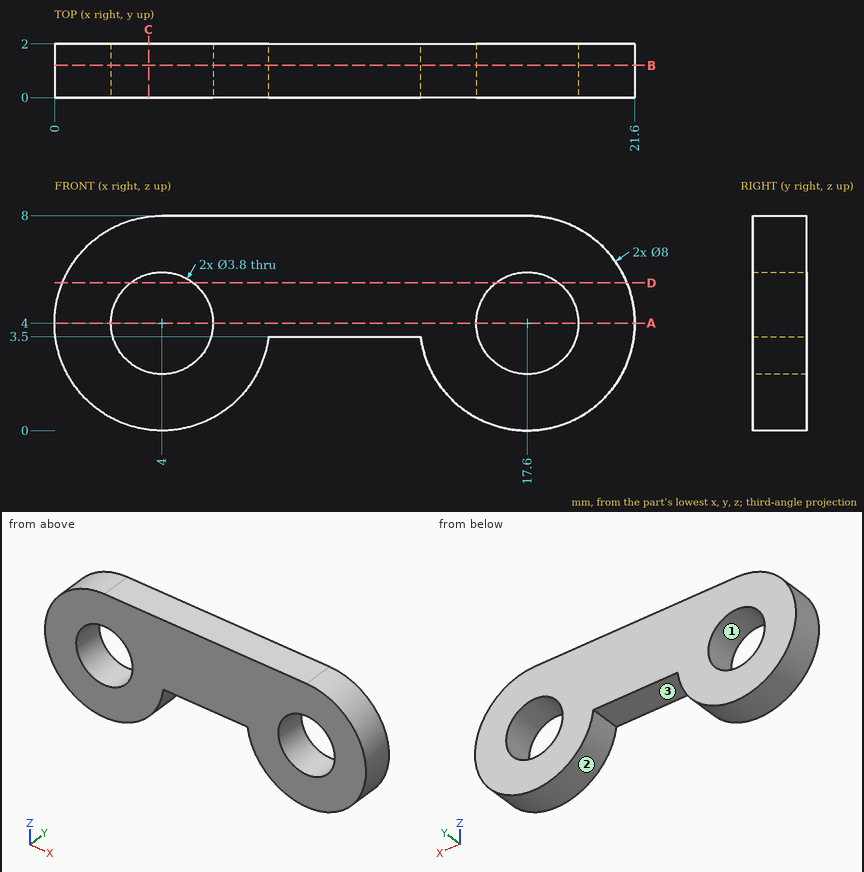
Can you work these out from the drawing? Everything is in mm from the part's minimum corner. Coordinates: 2 decimals unless noted, no trailing zeros. Loops run counter-clockwise (first coordinate to the right, second up) from the corner with the lowest first, then second, coordinate; pieces in that order, holes last. Notation, with made-up numbers: (41, 40.25) - (98, 40.25) arc R7 ccw to (98, 46.25) - close; hole circle Ø11 at (64.5, 33.5). An arc over 180 degrees is marked (long way). Put each result on its own line as item: value. Start each with the question number.
Item 1: Suppose I cut it at D-D (z = 5.5). Please give me the cut outline in (x, y).
Item 2: Suppose I cut it at A-A (z = 4). Please give me the cut outline in (x, y), and give its area (3 significant figures).
Item 3: If I drill on line 1 along X through (y, z) = (0.75, 4); line 2 along X through (y, z) = (1.5, 3.25); line 3 along X through (y, z) = (1.05, 5), over which ranges is the centre line in solid material (lowest first)?
Item 4: Suppose I cut it at C-C (x = 3.5). Please give me the cut outline in (y, z), and give its area (3 significant figures).
Item 5: For pin 1 (1 mm diameter, centred on y = 1.5, z = 1.5, fed in from -X), with a flat end and sliding along its axis, tell me the tip position at first contact or that it passes through.
Item 6: Suppose I cut it at B-B (y = 1.2). Please give me the cut outline in (x, z), and give its area (3 significant figures).
Item 7: If we mould it in two halves opening along Z, with no side actions, what happens to the marked faces 1, 2 and 3? For each: +Z half, -Z half, draft (parallel to the pull), parting line (faces both ways), or undercut.
Here are the results:
1. outline: (0.29, 0) - (2.83, 0) - (2.83, 2) - (0.29, 2) - close; (5.17, 0) - (16.43, 0) - (16.43, 2) - (5.17, 2) - close; (18.77, 0) - (21.31, 0) - (21.31, 2) - (18.77, 2) - close
2. outline: (0, 0) - (2.1, 0) - (2.1, 2) - (0, 2) - close; (5.9, 0) - (15.7, 0) - (15.7, 2) - (5.9, 2) - close; (19.5, 0) - (21.6, 0) - (21.6, 2) - (19.5, 2) - close
2. area: 28.0 mm²
3. line 1: 0 to 2.1, 5.9 to 15.7, 19.5 to 21.6
3. line 2: 0.07 to 2.25, 5.75 to 7.93, 13.67 to 15.85, 19.35 to 21.53
3. line 3: 0.13 to 2.38, 5.62 to 15.98, 19.22 to 21.47
4. outline: (0, 0.03) - (2, 0.03) - (2, 2.17) - (0, 2.17) - close; (0, 5.83) - (2, 5.83) - (2, 7.97) - (0, 7.97) - close
4. area: 8.54 mm²
5. pin 1: x = 0.54
6. outline: (4, 8) arc R4 ccw (long way) to (7.97, 3.5) - (13.63, 3.5) arc R4 ccw (long way) to (17.6, 8) - close; hole circle Ø3.8 at (4, 4); hole circle Ø3.8 at (17.6, 4)
6. area: 110 mm²
7. face 1: undercut
7. face 2: parting line
7. face 3: -Z half
